Work out the finished part from the listing and answer in its coordinate system (mm). A direction names the side the tool comes from. Round coordinates to 2 decimals unless told otherwise and drop trailing zeros. Order: outer loops, then holes, each group sorted by start corner. A loop starts at its lowest first (then second) coordinate and runs counter-clockwise, first axis right, second up. Notation, with made-up numbers: (67.25, 35) -> (75.25, 35) arc R24 cw to (75.25, 47) -> close; hole circle Ø5 at (-11.5, 76.5). An arc over 180 degrees is marked (long way). Use a Markdown table: item, result. Add a question column.
Item 1: A cutting plane is placed at B-B, the plane x = -57.5. Determine the outline of the cut face in (y, z) (3 decimals).
Item 2: A cutting plane is placed at D-D, the plane z = -52. Determine the outline of the cut face in (x, y), plus the area to 3 significant figures.
Item 3: A cutting plane is placed at C-C, the plane y = 9.75. Determine the outline of the cut face in (x, z) (1 decimal).
Item 4: Find the intervals of material crossed by L1, parallel to Z at x = -31, y = 2 (1 decimal); L2, parallel to X at y = 18, z = -42.5; L3, parallel to X at y = 4.5, z = -45.5, in increasing order. Write a range as [from, to].
Item 5: A cutting plane is placed at A-A, the plane z = -42.5. Determine the outline of the cut face in (x, y).
Item 6: A tool of negligible diameter and unlimited length cuts with its end or side. For faces 1 (the cylindrical face through (-22.914, 9.466, -46.06)), 2 (the flat face through (-46, 0, -50)), from which of +Z, -Z, +X, -X, +Y, -Y can it reach the whole face along a straight path? Write none if from no direction.
from build123d import *

# Parameters (mm, degrees)
SKETCH1_W           = 63.8
SKETCH1_H           = 31.8
SKETCH1_R           = 7.62
BOSS_EXTRUDE1_DEPTH = 19.2


with BuildPart() as part:
    # Sketch1 → Boss-Extrude1 (new body)
    with BuildSketch(Plane(origin=(0, 0, 0), x_dir=(1, 0, 0), z_dir=(0, 1, 0))):
        with Locations((-45.075543036, 45.955000213)):
            Rectangle(SKETCH1_W, SKETCH1_H)
        with Locations((-53.075543036, 45.955000213)):
            Circle(SKETCH1_R, mode=Mode.SUBTRACT)
        with BuildLine():
            Line((-40.375543036, 50.717500213), (-27.675543036, 50.717500213))
            ThreePointArc((-27.675543036, 50.717500213), (-22.913043036, 45.955000213), (-27.675543036, 41.192500213))
            Line((-27.675543036, 41.192500213), (-40.375543036, 41.192500213))
            ThreePointArc((-40.375543036, 41.192500213), (-45.138043036, 45.955000213), (-40.375543036, 50.717500213))
        make_face(mode=Mode.SUBTRACT)
    extrude(amount=BOSS_EXTRUDE1_DEPTH)


solid = part.part
Reported:
| question | item | result |
|---|---|---|
| 1 | outline | (0, -61.855) -> (19.2, -61.855) -> (19.2, -52.159) -> (0, -52.159) -> close; (0, -39.751) -> (19.2, -39.751) -> (19.2, -30.055) -> (0, -30.055) -> close |
| 2 | outline | (-76.98, 0) -> (-57.71, 0) -> (-57.71, 19.2) -> (-76.98, 19.2) -> close; (-48.44, 0) -> (-13.18, 0) -> (-13.18, 19.2) -> (-48.44, 19.2) -> close |
| 2 | area | 1,050 mm² |
| 3 | outline | (-77, -61.9) -> (-13.2, -61.9) -> (-13.2, -30.1) -> (-77, -30.1) -> close; hole circle Ø15.2 at (-53.1, -46); hole (-40.4, -50.7) -> (-27.7, -50.7) arc R4.8 ccw to (-27.7, -41.2) -> (-40.4, -41.2) arc R4.8 ccw to start |
| 4 | L1 | [-61.9, -50.7], [-41.2, -30.1] |
| 4 | L2 | [-76.98, -59.87], [-46.28, -43.65], [-24.4, -13.18] |
| 4 | L3 | [-76.98, -60.68], [-45.47, -45.12], [-22.93, -13.18] |
| 5 | outline | (-76.98, 0) -> (-59.87, 0) -> (-59.87, 19.2) -> (-76.98, 19.2) -> close; (-46.28, 0) -> (-43.65, 0) -> (-43.65, 19.2) -> (-46.28, 19.2) -> close; (-24.4, 0) -> (-13.18, 0) -> (-13.18, 19.2) -> (-24.4, 19.2) -> close |
| 6 | face 1 | +Y, -Y |
| 6 | face 2 | +Z, -Z, +X, -X, -Y |
